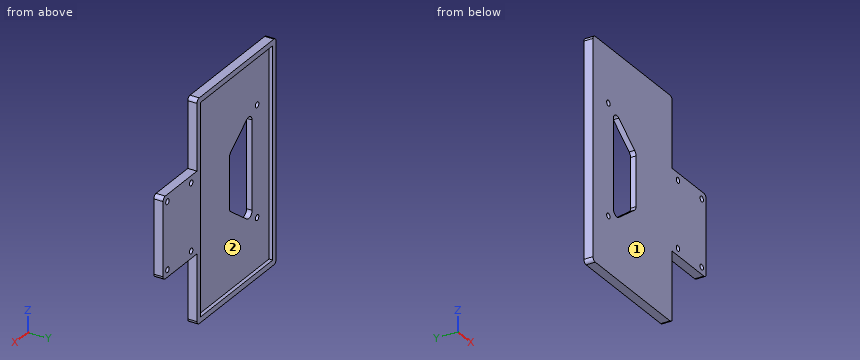
Autodesk Inventor part; units mm, degrees
ref_plane "YZ Plane" through (0, 0, 0) normal (1, 0, 0) x (0, 1, 0)
ref_plane "XZ Plane" through (0, 0, 0) normal (0, 1, 0) x (-1, 0, 0)
ref_plane "XY Plane" through (0, 0, 0) normal (0, 0, 1) x (1, 0, 0)
sketch "Sketch1" plane through (0, 0, 0) normal (0, 1, 0) x (-1, 0, 0)
  line L0 (0, 0) -> (70, 0)
  line L1 (70, 0) -> (70, -120)
  line L2 (70, -120) -> (0, -120)
  line L3 (0, -120) -> (0, 0)
  line L4 (0, -82) -> (-30, -82)
  line L5 (-30, -82) -> (-30, -38)
  line L6 (-30, -38) -> (0, -38)
  line L7 (0, -38) -> (0, -82)
  dimension "d0" = 70
  dimension "d1" = 120
  dimension "d2" = 44
  dimension "d3" = 30
  dimension "d4" = 38
  dimension "d5" = 38
extrude "Extrusion1" add sketch "Sketch1" along normal blind 5
sketch "Sketch2" plane through (0, 5, 0) normal (0, 1, 0) x (1, 0, 0)
  line L0 (-67, 3) -> (-3, 3)
  line L1 (-3, 3) -> (-3, 117)
  line L2 (-3, 117) -> (-67, 117)
  line L3 (-67, 117) -> (-67, 3)
  line L4 (-70, 0) -> (0, 0)
  line L5 (-70, 120) -> (-70, 0)
  line L6 (0, 120) -> (-70, 120)
  line L7 (0, 0) -> (0, 38)
  dimension "d8" = 3
  dimension "d10" = 3
  dimension "d12" = 3
  dimension "d13" = 3
extrude "Extrusion2" cut sketch "Sketch2" against normal blind 2
sketch "Sketch3" plane through (0, 3, 0) normal (0, 1, 0) x (1, 0, 0)
  line L0 (-52, 30) -> (-52, 90)
  line L1 (-52, 30) -> (-32, 45)
  line L2 (-32, 45) -> (-32, 75)
  line L3 (-32, 75) -> (-52, 90)
  line L4 (-67, 3) -> (-67, 117)
  line L5 (-3, 3) -> (-67, 3)
  line L6 (-67, 117) -> (-3, 117)
  circle A0 centre (-56.4262, 30) radius 1.5
  circle A1 centre (-56.4262, 90) radius 1.5
  point P0 (0, 0)
  dimension "d16" = 60
  dimension "d17" = 30
  dimension "d18" = 15
  dimension "d19" = 20
  dimension "d20" = 42
  dimension "d21" = 42
  dimension "d22" = 27
  dimension "d23" = 27
  dimension "d24" = 3
  dimension "d25" = 3
  dimension "d44" = 27
  dimension "d45" = 27
extrude "Extrusion3" cut sketch "Sketch3" against normal blind 10
fillet "Fillet1" radius 3 4 edges at (-52, 1.5, -30) (-32, 1.5, -45) (-32, 1.5, -75) (-52, 1.5, -90)
fillet "Fillet2" radius 2 6 edges at (0, 2.5, 0) (0, 2.5, -120) (-70, 2.5, -120) (-70, 2.5, 0) (30, 2.5, -38) (30, 2.5, -82)
sketch "Sketch4" plane through (0, 5, 0) normal (0, 1, 0) x (1, 0, 0)
  circle A0 centre (26.1, 41.9) radius 1.5
  line L0 (30, 40) -> (30, 80)
  line L1 (0, 38) -> (28, 38)
  circle A1 centre (26.1, 78.1) radius 1.5
  line L2 (28, 82) -> (0, 82)
  circle A2 centre (5.1, 41.9) radius 1.5
  circle A3 centre (5.1, 78.1) radius 1.5
  point P0 (0, 0)
  dimension "d30" = 3
  dimension "d31" = 3.9
  dimension "d32" = 3.9
  dimension "d33" = 3
  dimension "d34" = 3.9
  dimension "d35" = 3.9
  dimension "d36" = 3
  dimension "d37" = 21
  dimension "d38" = 3
  dimension "d39" = 21
  dimension "d40" = 3.9
  dimension "d41" = 3.9
extrude "Extrusion4" cut sketch "Sketch4" against normal blind 10
equation "\"d4\" = d5"
equation "\"d20\" = d21"
equation "\"d22\" = d23"
equation "\"d44\" = d22"
equation "\"d45\" = d22"
properties part number "drzaksolaru"
Geometry check sheet. Reference: the model listing, model coordinates, mm. Face numbers are marked on the shaded views. Round coordinates to 2 decimals unless told otherwise and drop trailing zeros. Loops run counter-clockwise (first coordinate to the right, second up) from the corner with the lowest first, then second, coordinate; pieces in that order, holes last.
Item 1: Mould release check, pull along X, two halves, no side actions. Record for the marked faces 1 and 2: pulls with the +X half, pulls with the -X half, needs draft (parallel to the pull), parting line crosses it, or undercut.
Item 2: Gauge pin test, flat ends, axial feed: pin 1 (1.8 mm diameter, centred on x = 5.1, z = -41.9, fed in from -Y); pin 2 (1 mm diameter, centred on x = 16.5, y = 1, fed in from -Z); pin 3 (3.5 mm diameter, centred on x = -56.43, z = -90, fed in from +Y). Record the tip position at first contact, or that the pin passes through.
Item 3: Cross-section at B-B on x = 5.1. Record the boundary of the cut face in (y, z).
Item 4: Cross-section at C-C on y = 3.9. Record the boundary of the cut face in (x, z), then the cut area to 3 significant figures.
Item 5: Cross-section at D-D on x = -20.5. Record the boundary of the cut face in (y, z).
Item 6: Thickness scan on line 1 (X direction, y = 3.4, z = -41.9); line 2 (Z direction, x = 26.1, y = 2.2); line 3 (X direction, y = 3.45, z = -63.5). Record the ranges inside material, lowest first.
Item 7: Cross-section at A-A on z = -57. Record the boundary of the cut face in (x, y).
Answer sheet:
1. face 1: needs draft
1. face 2: undercut
2. pin 1: passes through
2. pin 2: stops at z = -82
2. pin 3: stops at y = 3
3. outline: (0, -82) - (5, -82) - (5, -79.6) - (0, -79.6) - close; (0, -76.6) - (5, -76.6) - (5, -43.4) - (0, -43.4) - close; (0, -40.4) - (5, -40.4) - (5, -38) - (0, -38) - close
4. outline: (-70, -118) arc R2 ccw to (-68, -120) - (-2, -120) arc R2 ccw to (0, -118) - (0, -82) - (28, -82) arc R2 ccw to (30, -80) - (30, -40) arc R2 ccw to (28, -38) - (0, -38) - (0, -2) arc R2 ccw to (-2, 0) - (-68, 0) arc R2 ccw to (-70, -2) - close; hole (-67, -117) - (-3, -117) - (-3, -3) - (-67, -3) - close; hole circle Ø3 at (5.1, -78.1); hole circle Ø3 at (5.1, -41.9); hole circle Ø3 at (26.1, -78.1); hole circle Ø3 at (26.1, -41.9)
4. area: 2,390 mm2
5. outline: (0, -120) - (5, -120) - (5, -117) - (3, -117) - (3, -3) - (5, -3) - (5, 0) - (0, 0) - close
6. line 1: x = -70 to -67, -3 to 3.6, 6.6 to 24.6, 27.6 to 30
6. line 2: z = -82 to -79.6, -76.6 to -43.4, -40.4 to -38
6. line 3: x = -70 to -67, -3 to 30
7. outline: (-70, 0) - (-52, 0) - (-52, 3) - (-67, 3) - (-67, 5) - (-70, 5) - close; (-32, 0) - (30, 0) - (30, 5) - (-3, 5) - (-3, 3) - (-32, 3) - close
